Source: CAD feature listing. Evaluate the final solid. Frame: model axes, mm. A direction names the side the tool comes from. Coordinates: 2 decimals unless noted, no trailing zeros. Write each loop counter-clockwise with the first axis right and the second up, starting at its lowest first coordinate (ties: lowest second). Pieces come first, ordered by that corner, then holes. Notation, with made-up numbers: (62, 7) -> (118, 7) arc R26 ccw to (118, 28) -> close; hole circle Ø5 at (26.5, -23.5). An arc over 180 degrees is marked (long way). One line per item, written item: value. Start each with the question number.
1. Section query B-B, the plane z = 55. Output: boundary loops of the cut face in (x, y) (3 decimals), and give its area (3 significant figures).
2. Line query: line 1 (X direction, y = 6.5, z = 21) (3 decimals); line 2 (Y direction, x = -0.5, z = 141); line 3 (X direction, y = -12.5, z = 128). Output: solid intervals per line, ascending.
3. First-contact query: P1, Ø2, axis at x = -1, z = 37.5, coming from the -Y side (3 decimals); P2, Ø3.5, axis at x = -0.5, z = 18.5, coming from the +Y side (3 decimals); P3, Ø5, axis at x = -4, z = 89.5, coming from the +Y side. Flat tips, straight axial feed; report the tip coordinate or a pass-through.
4. Section query A-A, the plane z = 28.5. Output: boundary loops of the cut face in (x, y) (3 decimals).
5. Section query C-C, the plane y = -2. Output: boundary loops of the cut face in (x, z) (3 decimals).
6. Mould query, pull axis Y, two halves, no side actions, for faces 4 (the cylindrical face through (-7.807, -19.717, 141.499)), 5 (the flat face through (0, -8.245, 25)), 6 (the cylindrical face through (7.807, 12.717, 165.13)). Classes: released by +Y, released by -Y, zero draft, split by the parting line, or undercut.
7. Access query for faces 1 (the flat face through (-3.545, 0, 26)), 2 (the cylindrical face through (7.81, -14.96, 55.58)), 3 (the cylindrical face through (-7.81, -14.96, 57.13)). Directions: +Z, -Z, +X, -X, +Y, -Y. A direction counts if a zero-diameter tool reaches every point of the face in a straight line with its end or side. Return the directions, or none.
Autodesk Fusion 360 part; units mm, degrees
sketch "Schizzo1" plane through (0, 0, 0) normal (1, 0, 0) x (0, 1, 0)
  line L0 (18.245, 0) -> (18.245, 111.7185)
  line L1 (19.2011, 116.0715) -> (22.0439, 122.231)
  line L2 (23, 126.584) -> (23, 156.0021)
  line L3 (15.7382, 167.3516) -> (12.4928, 168.8495)
  line L4 (7.2545, 170) -> (0, 170)
  line L5 (18.245, 0) -> (0, 0)
  line L6 (0, 0) -> (0, 170) construction
  arc A0 (12.4928, 168.8495) -> (7.2545, 170) centre (7.2545, 157.5) ccw
  arc A1 (23, 156.0021) -> (15.7382, 167.3516) centre (10.5, 156.0021) ccw
  arc A2 (22.0439, 122.231) -> (23, 126.584) centre (12.6125, 126.584) ccw
  arc A3 (19.2011, 116.0715) -> (18.245, 111.7185) centre (28.6325, 111.7185) ccw
  line L7 (-18.245, 0) -> (0, 0)
  arc A4 (-18.245, 111.7185) -> (-19.2011, 116.0715) centre (-28.6325, 111.7185) ccw
  line L8 (-19.2011, 116.0715) -> (-22.0439, 122.231)
  arc A5 (-23, 126.584) -> (-22.0439, 122.231) centre (-12.6125, 126.584) ccw
  line L9 (-23, 126.584) -> (-23, 156.0021)
  arc A6 (-15.7382, 167.3516) -> (-23, 156.0021) centre (-10.5, 156.0021) ccw
  line L10 (-15.7382, 167.3516) -> (-12.4928, 168.8495)
  arc A7 (-7.2545, 170) -> (-12.4928, 168.8495) centre (-7.2545, 157.5) ccw
  line L11 (-7.2545, 170) -> (0, 170)
  line L12 (-18.245, 0) -> (-18.245, 111.7185)
  line L13 (-8.245, 0) -> (-8.245, 50)
  line L14 (-8.245, 50) -> (8.245, 50)
  line L15 (8.245, 50) -> (8.245, 0)
  point P0 (18.245, 114)
  point P1 (23, 124.3025)
  point P2 (23, 164)
  point P3 (10, 170)
  point P4 (0, 50)
  dimension "d1" = 170
  dimension "d2" = 18.245
  dimension "d3" = 56
  dimension "d4" = 10
  dimension "d5" = 23
  dimension "d6" = 23
  dimension "d7" = 6
  dimension "d8" = 12.5
  dimension "d9" = 12.5
  dimension "d10" = 10.3875
  dimension "d16" = 50
  dimension "d17" = 16.49
extrude "Estrusione1" add sketch "Schizzo1" along normal mid plane 21.84
extrude "Estrusione2" cut sketch "Schizzo1" along normal mid plane 7.09 contours L5 L7 L13 L14 L15
fillet "Raccordo1" radius 10.92 34 edges at (-10.92, -18.245, 55.8593) (-10.92, -18.4868, 113.9469) (-10.92, -20.6225, 119.1512) (-10.92, -22.7582, 124.3556) (-10.92, -23, 141.293) (-10.92, -21.0292, 162.739) (-10.92, -14.1155, 168.1005) (-10.92, -9.9361, 169.709) (-10.92, 0, 170) (-10.92, 9.9361, 169.709) (-10.92, 14.1155, 168.1005) (-10.92, 21.0292, 162.739) (-10.92, 23, 141.293) (-10.92, 22.7582, 124.3556) (-10.92, 20.6225, 119.1512) (-10.92, 18.4868, 113.9469) (-10.92, 18.245, 55.8593) (10.92, 18.245, 55.8593) (10.92, 18.4868, 113.9469) (10.92, 20.6225, 119.1512) (10.92, 22.7582, 124.3556) (10.92, 23, 141.293) (10.92, 21.0292, 162.739) (10.92, 14.1155, 168.1005) (10.92, 9.9361, 169.709) (10.92, 0, 170) (10.92, -9.9361, 169.709) (10.92, -14.1155, 168.1005) (10.92, -21.0292, 162.739) (10.92, -23, 141.293) (10.92, -22.7582, 124.3556) (10.92, -20.6225, 119.1512) (10.92, -18.4868, 113.9469) (10.92, -18.245, 55.8593)
chamfer "Smusso1" distance 1 angle 45 4 edges at (-3.545, 0, 0) (0, 8.245, 0) (3.545, 0, 0) (0, -8.245, 0)
chamfer "Smusso1" distance 1 angle 45 4 edges at (0, -18.245, 0) (10.92, 0, 0) (0, 18.245, 0) (-10.92, 0, 0)
equation "d1 = lunghezza_prolunga_freno"
equation "d2 = d17 / 2 + 10 mm"
equation "d5 = d6"
equation "d10 = -d2 * 2.5 + 56 mm"
equation "offset_incastro = 0.25 mm"
equation "larghezza_incastro = 16.24 mm"
equation "spessore_incastro = 6.84 mm"
equation "profondita_incastro = 50 mm"
equation "lunghezza_prolunga_freno = 170 mm"
equation "d16 = profondita_incastro"
equation "d17 = larghezza_incastro + offset_incastro"
equation "d18 = spessore_incastro + 15 mm"
equation "d20 = spessore_incastro + offset_incastro"
equation "d23 = d18 / 2"
Computed values:
1. outline: (-10.92, -7.327) arc R10.918 ccw to (-0.002, -18.245) -> (0.002, -18.245) arc R10.918 ccw to (10.92, -7.327) -> (10.92, 7.327) arc R10.918 ccw to (0.002, 18.245) -> (-0.002, 18.245) arc R10.918 ccw to (-10.92, 7.327) -> close
1. area: 695 mm²
2. line 1: x = -10.92 to -3.545, 3.545 to 10.92
2. line 2: y = -22.99 to 22.99
2. line 3: x = -10.91 to 10.91
3. P1: stops at y = -18.245
3. P2: stops at y = 18.245
3. P3: stops at y = 18.14
4. outline: (-10.92, -7.327) arc R10.918 ccw to (-0.002, -18.245) -> (0.002, -18.245) arc R10.918 ccw to (10.92, -7.327) -> (10.92, 7.327) arc R10.918 ccw to (0.002, 18.245) -> (-0.002, 18.245) arc R10.918 ccw to (-10.92, 7.327) -> close; hole (-3.545, -8.245) -> (3.545, -8.245) -> (3.545, 8.245) -> (-3.545, 8.245) -> close
5. outline: (-10.92, 1) -> (-9.92, 0) -> (-4.545, 0) -> (-3.545, 1) -> (-3.545, 50) -> (3.545, 50) -> (3.545, 1) -> (4.545, 0) -> (9.92, 0) -> (10.92, 1) -> (10.92, 159.082) arc R10.918 ccw to (0.002, 170) -> (-0.002, 170) arc R10.918 ccw to (-10.92, 159.082) -> close
6. face 4: released by -Y
6. face 5: undercut
6. face 6: released by +Y
7. face 1: -Z
7. face 2: -Z, +X, -Y
7. face 3: -Z, -X, -Y
